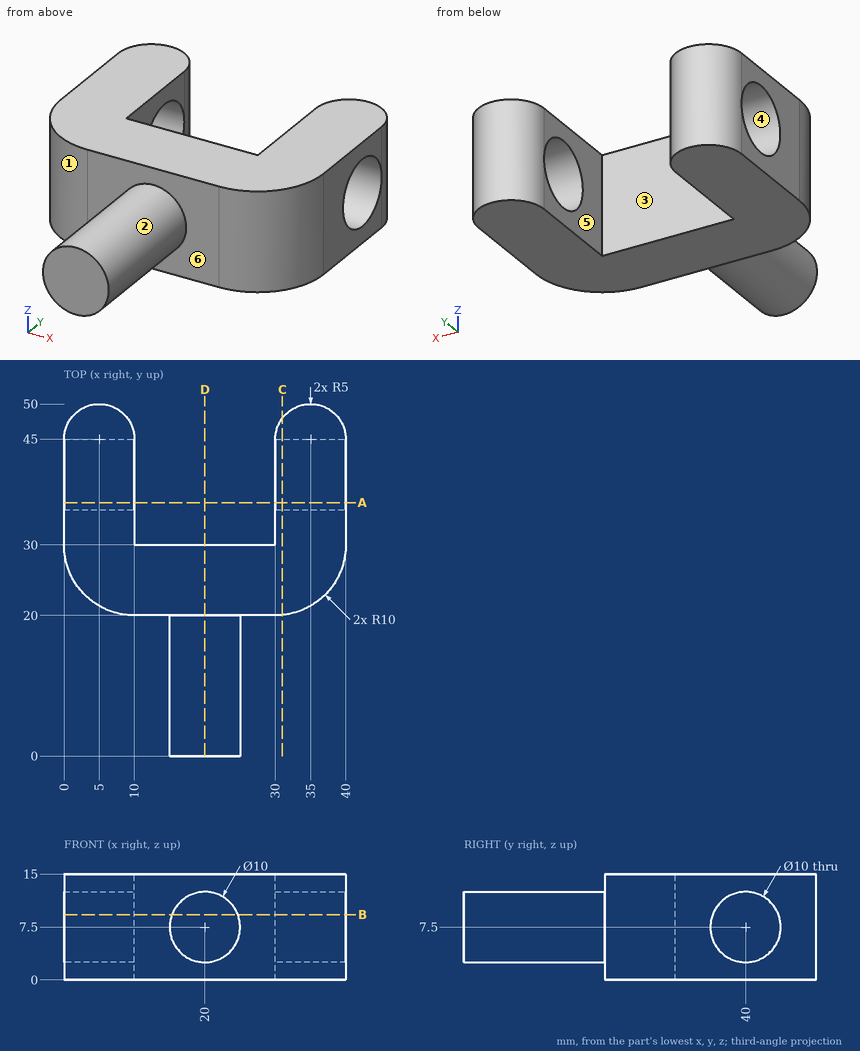
Study the drawing (mm; zero at the part's minimum x, y, z) and answer. A direction names the side the tool comes from. Give positions to 0.01 mm unless a question says otherwise; leave off trailing zeros. Loops run counter-clockwise (first coordinate to the right, second up) from the corner with the lowest first, then second, coordinate; pieces in that order, holes last. Notation, with made-up numbers: (80.25, -19.75) - (98.25, -19.75) arc R15 ccw to (98.25, -4.75) - close; hole circle Ø7 at (-16.75, 18.5). An arc over 180 degrees is marked (long way). One line per question, with ' | ' between items.
(1) Straight lines are drawn through the part: probe 1 along X at (y, z) = (35, 4.5); probe 2 along Z at (x, y) = (33.5, 40); probe 3 along Y at (x, z) = (28.5, 13). For each, find the intervals that lie inside material, in ascending order.
Recorded:
probe 1: x = 0 to 10, 30 to 40 | probe 2: z = 0 to 2.5, 12.5 to 15 | probe 3: y = 20 to 30
(2) The mould has two halves that part along Y. Classify the marked faces 4, 5 and 6: +Y half, -Y half, draft (parallel to the pull), parting line (faces both ways), or undercut.
Recorded:
face 4: undercut | face 5: draft | face 6: -Y half
(3) The part is cut by section B-B (z = 9.25). Write down the section's boundary in (x, y).
Recorded:
outline: (0, 30) arc R10 ccw to (10, 20) - (15.32, 20) - (15.32, 0) - (24.68, 0) - (24.68, 20) - (30, 20) arc R10 ccw to (40, 30) - (40, 35.32) - (30, 35.32) - (30, 30) - (10, 30) - (10, 35.32) - (0, 35.32) - close; (0, 44.68) - (10, 44.68) - (10, 45) arc R5 ccw to (0, 45) - close; (30, 44.68) - (40, 44.68) - (40, 45) arc R5 ccw to (30, 45) - close
(4) Each of these flat-tipped pins is pushed along its axis until it touches: pin 1 Ø6 at (x, z) = (12, 4.5) entering from +Y; pin 2 Ø1 at (y, z) = (26.5, 11.5) entering from -X; pin 3 Ø7.5 at (x, z) = (16.5, 7.5) entering from +Y; pin 4 Ø8 at (x, z) = (16.5, 11.5) entering from -Y. Where does it stop, or does it pass through?
Recorded:
pin 1: stops at y = 48 | pin 2: stops at x = 0.46 | pin 3: stops at y = 30 | pin 4: stops at y = 0
(5) The part is cut by section D-D (x = 20). Write down the section's boundary in (y, z).
Recorded:
outline: (0, 2.5) - (20, 2.5) - (20, 0) - (30, 0) - (30, 15) - (20, 15) - (20, 12.5) - (0, 12.5) - close
(6) The part is cut by section C-C (x = 31). Write down the section's boundary in (y, z), then the cut area to 3 significant figures.
Recorded:
outline: (20.05, 0) - (48, 0) - (48, 15) - (20.05, 15) - close; hole circle Ø10 at (40, 7.5) | area: 341 mm²
(7) A tool of negligible diameter and unlimited length cuts with its end or side. For the marked faces 1, 2 and 3, from which of +Z, -Z, +X, -X, +Y, -Y can it reach the whole face along a straight path? Write none if from no direction.
Recorded:
face 1: +Z, -Z, -X, -Y | face 2: -Y | face 3: +Z, -Z, +Y
(8) The part is cut by section A-A (y = 36). Write down the section's boundary in (x, z), then the cut area to 3 significant figures.
Recorded:
outline: (0, 0) - (10, 0) - (10, 4.5) - (0, 4.5) - close; (0, 10.5) - (10, 10.5) - (10, 15) - (0, 15) - close; (30, 0) - (40, 0) - (40, 4.5) - (30, 4.5) - close; (30, 10.5) - (40, 10.5) - (40, 15) - (30, 15) - close | area: 180 mm²
